Source: three-view drawing plus pictorial views. Frame: mm from the lowest corner of the part. A direction names the side the tool comes from. Coordinates: 2 decimals unless noted, no trailing zeros. Order: outer loops, then holes, each group sorted by start corner. A loop starts at its lowest first (then second) coordinate and runs counter-clockwise, first axis right, second up. Notation, with made-up numbers: (-23, -10) -> (-6, -10) arc R25 cw to (-6, 13) -> close; hole circle Ø6 at (75.5, 17). An arc over 180 degrees is marked (long way). One line per question, with ' | ' between items.
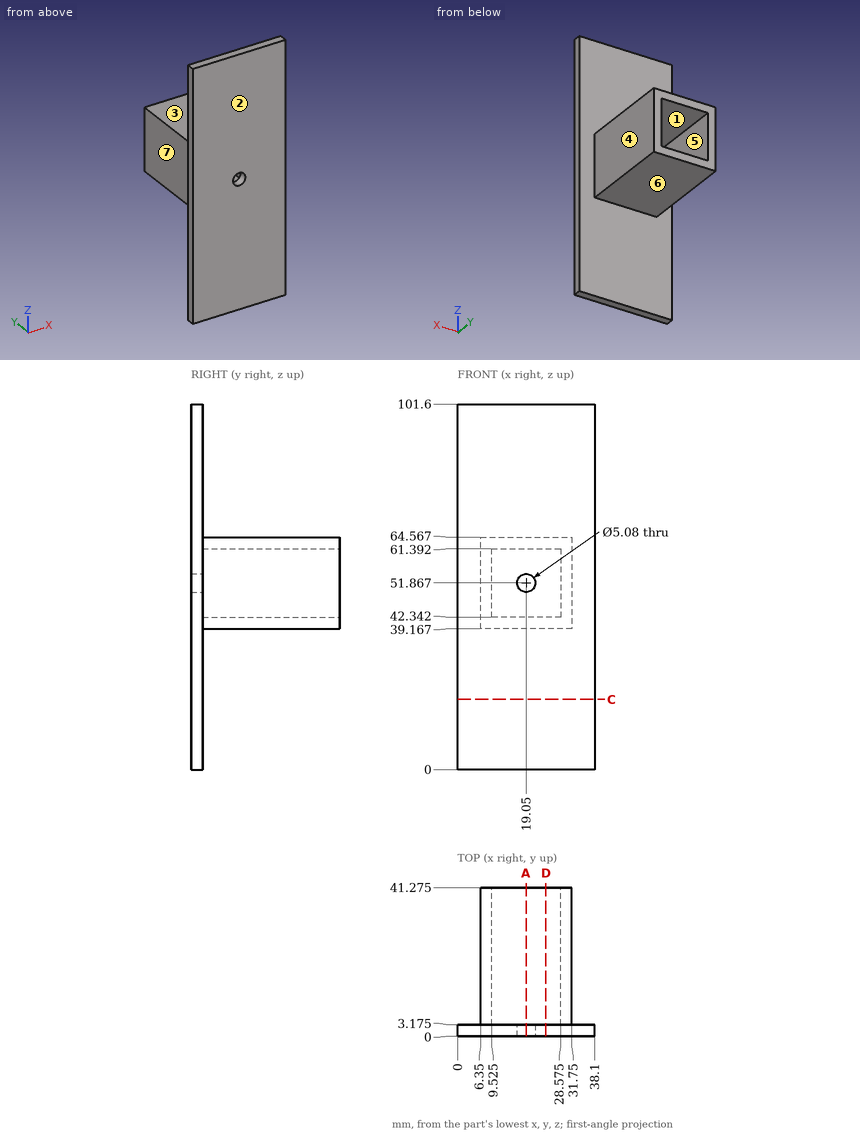
1. Mould query, pull axis X, two halves, no side actions, for the marked faces 5, 6 and 7. Classes: released by +X, released by -X, zero draft, split by the parting line, or undercut.
Recorded:
face 5: undercut | face 6: zero draft | face 7: released by -X
2. Ray query, line 1 (Z direction, x = 23.5, y = 20.5); line 2 (Z direction, x = 19.05, y = 2.2); line 3 (X direction, y = 35.5, z = 61) (3 decimals). Return the intervals inside material, ascending. Write a range as [from, to].
Recorded:
line 1: z = [39.17, 42.34], [61.39, 64.57] | line 2: z = [0, 49.33], [54.41, 101.6] | line 3: x = [6.35, 9.525], [28.575, 31.75]
3. Cut plane D-D, the plane x = 24.5. Return loops of the section in (y, z) (1 decimal).
Recorded:
outline: (0, 0) -> (3.2, 0) -> (3.2, 39.2) -> (41.3, 39.2) -> (41.3, 42.3) -> (3.2, 42.3) -> (3.2, 61.4) -> (41.3, 61.4) -> (41.3, 64.6) -> (3.2, 64.6) -> (3.2, 101.6) -> (0, 101.6) -> close
4. Pin query (flat end, axial travel): pin 1 Ø1.5 at (x, y) = (19.5, 26) entering from +Z; pin 2 Ø15 at (y, z) = (28.5, 49.5) entering from -X; pin 3 Ø7.5 at (x, y) = (19, 20) entering from -Z. Return the tip coordinate at first contact, or that it passes through.
Recorded:
pin 1: stops at z = 64.57 | pin 2: stops at x = 6.35 | pin 3: stops at z = 39.17
5. Cut plane C-C, the plane z = 19.5. Return loops of the section in (x, y) (3 decimals).
Recorded:
outline: (0, 0) -> (38.1, 0) -> (38.1, 3.175) -> (0, 3.175) -> close
6. Cut plane A-A, the plane x = 19.05. Return loops of the section in (y, z) (1 decimal).
Recorded:
outline: (0, 0) -> (3.2, 0) -> (3.2, 39.2) -> (41.3, 39.2) -> (41.3, 42.3) -> (3.2, 42.3) -> (3.2, 49.3) -> (0, 49.3) -> close; (0, 54.4) -> (3.2, 54.4) -> (3.2, 61.4) -> (41.3, 61.4) -> (41.3, 64.6) -> (3.2, 64.6) -> (3.2, 101.6) -> (0, 101.6) -> close
7. Access query for the marked faces 1, 2, 3 and 4. Directions: +Z, -Z, +X, -X, +Y, -Y. A direction counts if a zero-diameter tool reaches every point of the face in a straight line with its end or side. Return the directions, or none.
Recorded:
face 1: +Y | face 2: +Z, -Z, +X, -X, -Y | face 3: +Z, +X, -X, +Y | face 4: +Z, -Z, +X, +Y
